The model under review builds one solid part; all positions refer to its coordinate system, in mm. Face numbers are marked on the shaded views. A direction names the side the tool comes from. Coordinates: 2 decimals unless noted, no trailing zeros. Loops run counter-clockwise (first coordinate to the right, second up) from the corner with the lowest first, then second, coordinate; pieces in that order, holes last. Notation, with made-up numbers: (67, -23) - (74, -23) arc R32 ccw to (74, 15) - close; hole circle Ø2 at (57, 23.25). An arc over 180 degrees is marked (long way). One line per item, written item: value. Start each with the question number.
1. We need section B-B, the plane z = -13.5. Give the boundary of the cut face in (x, y), then the cut area to 3 significant figures.
2. We need section C-C, the plane x = 13. Give the boundary of the cut face in (y, z).
3. We need section A-A, the plane x = 10.25. Give the boundary of the cut face in (y, z), then the cut area to 3 significant figures.
4. To check wall thickness, follow line 1 (Z direction, x = 3.25, y = 1.6); line 2 (Z direction, x = 14.75, y = 1.8); line 3 (X direction, y = 2, z = -13.75). State the ranges of each line that lie inside material, in increasing order.
5. We need section D-D, the plane z = -5.25. Give the boundary of the cut face in (x, y).
6. For the marked faces 1 and 2, list the 3-axis set-ups (+Z, -Z, +X, -X, +Y, -Y) from which the entire face can be reached by the end or side of a thin tool; tool diameter is ignored.
7. Insertion check: P1, Ø0.6, axis at x = 1.5, y = 2, coming from the +Z side; P2, Ø0.6, axis at x = 8, y = 2, coming from the +Z side; P3, Ø1, axis at y = 2, z = -5, coming from the -X side. Each pin has a flat end and moves straight along its axis. Give the tip position at first contact, or say it passes through.
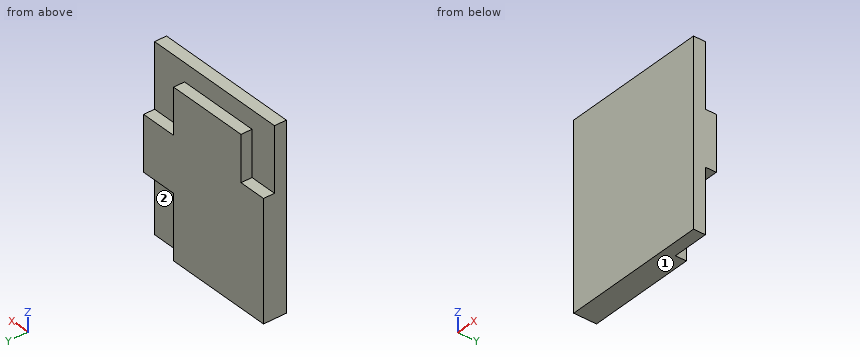
from build123d import *

# Parameters (mm, degrees)
SKETCH1_W           = 16
SKETCH1_H           = 20
BOSS_EXTRUDE1_DEPTH = 1.3
BOSS_EXTRUDE2_DEPTH = 1.2


with BuildPart() as part:
    # Sketch1 → Boss-Extrude1 (new body)
    with BuildSketch(Plane(origin=(0, 0, 0), x_dir=(1, 0, 0), z_dir=(0, 1, 0))):
        with Locations((8, 10)):
            Rectangle(SKETCH1_W, SKETCH1_H)
    extrude(amount=BOSS_EXTRUDE1_DEPTH)

    # Sketch2 → Boss-Extrude2 (add)
    with BuildSketch(Plane(origin=(0, 1.3, 0), x_dir=(1, 0, 0), z_dir=(0, 1, 0))):
        Polygon((3, 7), (3, 2), (12, 2), (12, 7), (16, 7), (16, 13), (12, 13), (12, 20), (0, 20), (0, 7), align=None)
    extrude(amount=BOSS_EXTRUDE2_DEPTH)


solid = part.part
Findings below:
1. outline: (0, 0) - (16, 0) - (16, 1.3) - (12, 1.3) - (12, 2.5) - (0, 2.5) - close
1. area: 35.2 mm2
2. outline: (0, -20) - (1.3, -20) - (1.3, -13) - (2.5, -13) - (2.5, -7) - (1.3, -7) - (1.3, 0) - (0, 0) - close
3. outline: (0, -20) - (2.5, -20) - (2.5, -2) - (1.3, -2) - (1.3, 0) - (0, 0) - close
3. area: 47.6 mm2
4. line 1: -20 to -2
4. line 2: -13 to -7
4. line 3: 0 to 12
5. outline: (0, 0) - (16, 0) - (16, 1.3) - (12, 1.3) - (12, 2.5) - (3, 2.5) - (3, 1.3) - (0, 1.3) - close
6. face 1: -Z, +X, -X, +Y, -Y
6. face 2: -Z, +X, +Y
7. P1: z = -7
7. P2: z = -2
7. P3: x = 3
